Work out the finished part from the listing and answer in its coordinate system (mm). A direction names the side the tool comes from. Give positions to 0.01 mm unless a question says otherwise; leave off trailing zeros. Order: outer loops, then holes, each group sorted by start corner. A loop starts at its lowest first (then second) coordinate and runs counter-clockwise, first axis right, second up.
```python
from build123d import *

# Parameters (mm, degrees)
SKETCH1_R           = 9
EXTRUDE1_DEPTH      = 62.5
CHAMFER1_SIZE       = 1.35
SKETCH3_W           = 6
SKETCH3_H           = 3.5
EXTRUDE2_DEPTH      = 63.5
EXTRUDE2_DEPTH_BACK = 63.5


with BuildPart() as part:
    # Sketch1 → Extrude1 (new body, symmetric)
    with BuildSketch(Plane.XY):
        Circle(SKETCH1_R)
    extrude(amount=EXTRUDE1_DEPTH, both=True)

    # Chamfer1
    chamfer1_edges = [part.edges().sort_by_distance(p)[0] for p in [
        (-9, 0, -62.5),
        (-9, 0, 62.5),
    ]]
    chamfer(chamfer1_edges, length=CHAMFER1_SIZE)

    # Sketch3 → Extrude2 (cut, two sides)
    with BuildSketch(Plane.XY) as extrude2_sk:
        with Locations((0, 7.25)):
            Rectangle(SKETCH3_W, SKETCH3_H)
    extrude(amount=EXTRUDE2_DEPTH, mode=Mode.SUBTRACT)
    extrude(extrude2_sk.sketch, amount=-EXTRUDE2_DEPTH_BACK, mode=Mode.SUBTRACT)


solid = part.part
```
1. Given P1, Ø5, axis at y = 6, z = 34.5, coming from the -X side; P2, Ø6, axis at x = -4, z = 39, coming from the -Y side; P3, Ø3, axis at y = -4, z = 35.5, coming from the -X side, each flat-ended and moving along its own axis, determine where each tip first touches the part or whether it passes through.
Findings below:
P1: stops at x = -8.29
P2: stops at y = -8.94
P3: stops at x = -8.65
2. The mould has two halves that part along X. Classify faces 3 (the face through (-0.308, -7.859, 62.284)), 4 (the face through (0, 0, 62.5)), 5 (the face through (0, 5.5, -1)): pulls with the +X half, pulls with the -X half, needs draft (parallel to the pull), parting line crosses it, or undercut.
Findings below:
face 3: parting line crosses it
face 4: needs draft
face 5: undercut
3. Which of the six approach directions +Z, -Z, +X, -X, +Y, -Y give full straight-line access (tool end or side, diameter ignored) to faces 1 (the face through (-3, 7, 1)), 2 (the face through (0, 0, -62.5))?
Findings below:
face 1: +Z, -Z, +Y
face 2: -Z, +X, -X, +Y, -Y
4. Straight lines are drawn through the part: probe 1 along X at (y, z) = (6.25, -48); probe 2 along Y at (x, z) = (-4.75, 3); probe 3 along X at (y, z) = (-0.5, 56.5). For each, find the intervals that lie inside material, in ascending order.
Findings below:
probe 1: x = -6.48 to -3, 3 to 6.48
probe 2: y = -7.64 to 7.64
probe 3: x = -8.99 to 8.99
5. The part is cut by section A-A (x = 0). Write down the section's boundary in (y, z), then the cut area to 3 significant figures.
Findings below:
outline: (-9, -61.15) - (-7.65, -62.5) - (5.5, -62.5) - (5.5, 62.5) - (-7.65, 62.5) - (-9, 61.15) - close
area: 1,810 mm2
6. The part is cut by section B-B (z = 17). Write down the section's boundary in (x, y), then the cut area to 3 significant figures.
Findings below:
outline: (-3, 5.5) - (-3, 8.49) arc R9 ccw (long way) to (3, 8.49) - (3, 5.5) - close
area: 234 mm2
